Check sheet for the modelled part. Datum: model origin and axes. Units: mm. Face numbers are marked on the shaded views. A direction names the side the tool comes from. Give positions to 0.01 mm unless a question says otherwise; leave off trailing zeros. Order: outer loops, then holes, each group sorted by start corner. A loop starts at its lowest first (then second) coordinate and runs counter-clockwise, first axis right, second up. Notation, with made-up numbers: (89, 75.5) -> (145, 75.5) arc R11 cw to (145, 81.5) -> close; hole circle Ø5 at (74, 20). An arc over 180 degrees is marked (long way). Write each question's results on one line, items separated by ' | '.
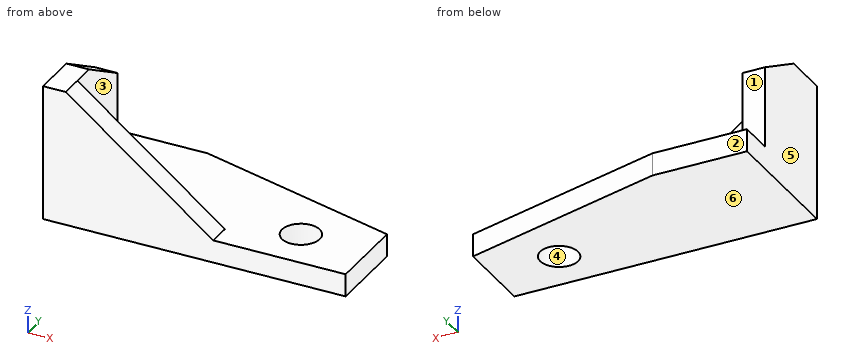
from build123d import *

# Parameters (mm, degrees)
SKETCH_1_R      = 5
EXTRUDE_1_DEPTH = 6
EXTRUDE_2_DEPTH = 6
EXTRUDE_3_DEPTH = 6


with BuildPart() as part:
    # 草圖1 → 填料-伸長1 (new body)
    with BuildSketch(Plane.XY):
        Polygon((0, 0), (80, 0), (80, 21.262794416), (25, 36), (0, 36), align=None)
        with Locations((62, 12)):
            Circle(SKETCH_1_R, mode=Mode.SUBTRACT)
    extrude(amount=-EXTRUDE_1_DEPTH)

    # 草圖2 → 填料-伸長2 (add)
    with BuildSketch(Plane(origin=(0, 0, 0), x_dir=(0, 0, -1), z_dir=(1, 0, 0))):
        Polygon((0, 0), (-30, 0), (-30, 12), (-21.492830392, 26.73484999), (0, 26.73484999), align=None)
    extrude(amount=EXTRUDE_2_DEPTH)

    # 草圖3 → 填料-伸長3 (add)
    with BuildSketch(Plane(origin=(0, 0, 0), x_dir=(1, 0, 0), z_dir=(0, 1, 0))):
        Polygon((0, 0), (45, 0), (6, -30), (0, -30), align=None)
    extrude(amount=EXTRUDE_3_DEPTH)


solid = part.part
1. Section check B-B on x = 62. Record the cut outline in (y, z).
Verdict:
outline: (0, -6) -> (7, -6) -> (7, 0) -> (0, 0) -> close; (17, -6) -> (26.09, -6) -> (26.09, 0) -> (17, 0) -> close
2. Gauge pin test, flat ends, axial feed: pin 1 Ø12 at (y, z) = (26.5, 20) entering from +X; pin 2 Ø8 at (x, y) = (47.5, 25.5) entering from +Z; pin 3 Ø9 at (x, z) = (20.5, 21) entering from +Y; pin 4 Ø1.5 at (y, z) = (28, 5) entering from +X. Record the tip position at first contact, or that the pin passes through.
Verdict:
pin 1: stops at x = 6 | pin 2: stops at z = 0 | pin 3: stops at y = 6 | pin 4: passes through
3. Mould release check, pull along X, two halves, no side actions. Record for the marked faces 3, 4, 5 and 6: +X half, -X half, draft (parallel to the pull), parting line (faces both ways), or undercut.
Verdict:
face 3: +X half | face 4: undercut | face 5: -X half | face 6: draft
4. Section check C-C on z = 19.5. Record the cut outline in (x, y).
Verdict:
outline: (0, 0) -> (19.65, 0) -> (19.65, 6) -> (6, 6) -> (6, 26.73) -> (0, 26.73) -> close
5. Material ranges on probe 1 along Z at (x, y) = (72, 11); probe 2 along X at (y, z) = (7, 5.5); probe 3 along Y at (x, z) = (62, -2.55), recorded low to high. Write a range as from..to.
Verdict:
probe 1: z = -6..0 | probe 2: x = 0..6 | probe 3: y = 0..7, 17..26.09
6. Access from +Z, -Z, +X, -X, +Y, -Y to the whole of each face (thin tool, end or side, straight path). Record for the marked faces 1 and 2.
Verdict:
face 1: +Z, +X, -X, +Y | face 2: +Z, -Z, +X, -X, +Y
7. Section check D-D on y = 24. Record the cut outline in (x, z), then the cut area to 3 significant figures.
Verdict:
outline: (0, -6) -> (69.78, -6) -> (69.78, 0) -> (6, 0) -> (6, 23.07) -> (0, 23.07) -> close | area: 557 mm^2
8. Section check A-A on z = -1. Record the cut outline in (x, y), then the cut area to 3 significant figures.
Verdict:
outline: (0, 0) -> (80, 0) -> (80, 21.26) -> (25, 36) -> (0, 36) -> close; hole circle Ø10 at (62, 12) | area: 2,400 mm^2
